Could you check a few things on this model? Use its own coordinates, in mm. Face numbers are marked on the shaded views. A direction names the side the tool comes from. Coordinates: 2 decimals unless noted, no trailing zeros. Order: outer loops, then holes, each group sorted by start corner. A loop starts at its lowest first (then second) coordinate and runs counter-clockwise, first axis right, second up. Notation, with made-up numbers: (-37.75, -29.75) - (-22.75, -29.75) arc R14 cw to (-22.75, -9.75) - close; hole circle Ø3 at (26.25, 61.25). An arc over 180 degrees is marked (long way). One line per item, written item: value. Start each with the question number.
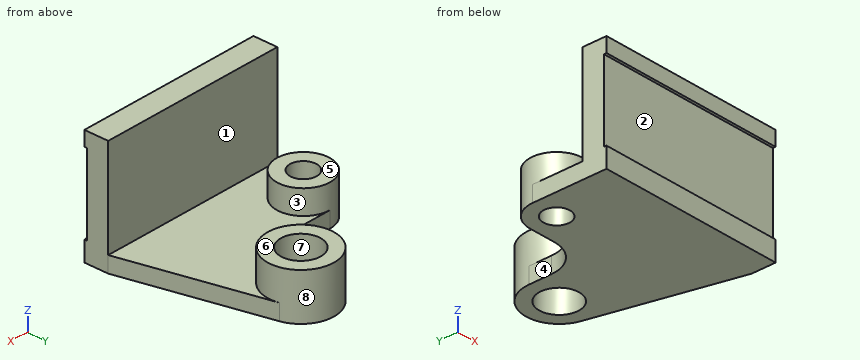
from build123d import *

# Parameters (mm, degrees)
SKETCH1_W           = 140
SKETCH1_H           = 18
BOSS_EXTRUDE1_DEPTH = 86
BOSS_EXTRUDE2_DEPTH = 12
SKETCH1_4_R         = 25
SKETCH1_4_R_2       = 15
BOSS_EXTRUDE3_DEPTH = 35
SKETCH1_5_R         = 20
SKETCH1_5_R_2       = 10
BOSS_EXTRUDE4_DEPTH = 30
CUT_EXTRUDE1_REACH  = 219.819
SKETCH4_W           = 60
SKETCH4_H           = 2


with BuildPart() as part:
    # Sketch1 → Boss-Extrude1 (new body)
    with BuildSketch(Plane.XY):
        with Locations((-20, 9)):
            Rectangle(SKETCH1_W, SKETCH1_H)
    extrude(amount=BOSS_EXTRUDE1_DEPTH)

    # Sketch1_3 → Boss-Extrude2 (add)
    with BuildSketch(Plane.XY):
        with BuildLine():
            Line((-90, 18), (50, 18))
            Line((50, 18), (24.294494718, 123.897247359))
            ThreePointArc((24.294494718, 123.897247359), (24.822997079, 120.969649142), (25, 118))
            ThreePointArc((25, 118), (0, 93), (-25, 118))
            Line((-25, 118), (-25, 101))
            ThreePointArc((-25, 101), (-32.32233047, 83.32233047), (-50, 76))
            Line((-50, 76), (-70, 76))
            ThreePointArc((-70, 76), (-55.857864376, 70.142135624), (-50, 56))
            ThreePointArc((-50, 56), (-70, 36), (-90, 56))
            Line((-90, 56), (-90, 18))
        make_face()
    extrude(amount=BOSS_EXTRUDE2_DEPTH)

    # Sketch1_4 → Boss-Extrude3 (add)
    with BuildSketch(Plane.XY):
        with Locations(Location((0, 118, 0), (0, 0, 180))):
            Circle(SKETCH1_4_R)
        with Locations((0, 118)):
            Circle(SKETCH1_4_R_2, mode=Mode.SUBTRACT)
    extrude(amount=BOSS_EXTRUDE3_DEPTH)

    # Sketch1_5 → Boss-Extrude4 (add)
    with BuildSketch(Plane.XY):
        with Locations(Location((-70, 56, 0), (0, 0, 180))):
            Circle(SKETCH1_5_R)
        with Locations((-70, 56)):
            Circle(SKETCH1_5_R_2, mode=Mode.SUBTRACT)
    extrude(amount=BOSS_EXTRUDE4_DEPTH)

    # Sketch4 → Cut-Extrude1 (cut, up to next)
    with BuildSketch(Plane(origin=(50, 0, 0), x_dir=(0, 0, -1), z_dir=(1, 0, 0)), mode=Mode.PRIVATE) as cut_extrude1_sk1:
        with Locations((-45, 1)):
            Rectangle(SKETCH4_W, SKETCH4_H)
    cut_extrude1_tool1 = extrude(cut_extrude1_sk1.sketch, amount=-CUT_EXTRUDE1_REACH, mode=Mode.PRIVATE) & part.part
    add(cut_extrude1_tool1.solids().sort_by_distance((50, 1, 45))[0], mode=Mode.SUBTRACT)


solid = part.part
Q1. I want a section at B-B on x = 0. Please give me the cut outline in (y, z).
Q2. We'd pull the mould along X, two halves only. Please class the marked faces 6, 7 and 8: +X half, -X half, draft (parallel to the pull), parting line (faces both ways), or undercut.
Q3. I'm going to push flat-ended pins straight in: pin 1 (4 mm diameter, centred on x = -61.5, y = 39, fed in from -Z); pin 2 (12 mm diameter, centred on x = -66.5, y = 63, fed in from +Z); pin 3 (6 mm diameter, centred on y = 112.5, z = 7, fed in from -X); pin 4 (1 mm diameter, centred on y = 55.5, z = 24.5, fed in from +X). Where does each tip first touch, or does it pass through?
Q4. I want a section at A-A on z = 24. Please give me the cut outline in (x, y).
Q5. I want a section at D-D on x = -58. Please give me the cut outline in (y, z).
Q6. If I drill on L1, parallel to Y at x = 0, z = 27.5; L2, parallel to Y at x = 0, z = 11; L3, parallel to Y at x = -70, z = 20, over which ranges is the centre line in solid material (lowest first)?
Q7. I want a section at C-C on y = 40. Please give me the cut outline in (x, z).
Q8. Which directions (+Z, -Z, +X, -X, +Y, -Y) give clear straight access to the entire face, cutting with the end or side of a thin tool? Please do the marked faces 1, 2, 3, 4 and 5.
Values follow:
1. outline: (0, 0) - (103, 0) - (103, 35) - (93, 35) - (93, 12) - (18, 12) - (18, 86) - (0, 86) - (0, 75) - (2, 75) - (2, 15) - (0, 15) - close; (133, 0) - (143, 0) - (143, 35) - (133, 35) - close
2. face 6: draft
2. face 7: undercut
2. face 8: parting line
3. pin 1: stops at z = 0
3. pin 2: stops at z = 30
3. pin 3: stops at x = -25
3. pin 4: stops at x = -50
4. outline: (-90, 2) - (50, 2) - (50, 18) - (-90, 18) - close; circle Ø40 at (-70, 56); circle Ø50 at (0, 118); hole circle Ø20 at (-70, 56); hole circle Ø30 at (0, 118)
5. outline: (0, 0) - (76, 0) - (76, 12) - (72, 12) - (72, 30) - (40, 30) - (40, 12) - (18, 12) - (18, 86) - (0, 86) - (0, 75) - (2, 75) - (2, 15) - (0, 15) - close
6. L1: y = 2 to 18, 93 to 103, 133 to 143
6. L2: y = 0 to 103, 133 to 143
6. L3: y = 2 to 18, 36 to 46, 66 to 76
7. outline: (-90, 0) - (44.66, 0) - (44.66, 12) - (-58, 12) - (-58, 30) - (-82, 30) - (-82, 12) - (-90, 12) - close
8. face 1: +Z, +X, -X
8. face 2: +X, -X, -Y
8. face 3: +Z
8. face 4: +Z, -Z, -X, +Y
8. face 5: +Z, +X, -X, +Y
